Autodesk Inventor part; units mm, degrees
ref_plane "YZ Plane" through (0, 0, 0) normal (1, 0, 0) x (0, 1, 0)
ref_plane "XZ Plane" through (0, 0, 0) normal (0, 1, 0) x (-1, 0, 0)
ref_plane "XY Plane" through (0, 0, 0) normal (0, 0, 1) x (1, 0, 0)
sketch "Sketch1" plane through (0, 0, 0) normal (0, 0, 1) x (1, 0, 0)
  line L0 (0, 0) -> (35, 0)
  line L1 (35, 0) -> (35, 4.5)
  line L2 (35, 4.5) -> (4.5, 4.5)
  line L3 (4.5, 4.5) -> (4.5, 35)
  line L4 (4.5, 35) -> (0, 35)
  line L5 (0, 35) -> (0, 0)
  dimension "d0" = 35
  dimension "d1" = 35
  dimension "d2" = 4.5
  dimension "d3" = 4.5
extrude "Extrusion1" add sketch "Sketch1" along normal mid plane 28
sketch "Sketch2" plane through (0, 0, 14) normal (0, 0, 1) x (1, 0, 0)
  line L0 (0, 0) -> (35, 0)
  line L1 (35, 0) -> (35, 4.5)
  line L2 (35, 4.5) -> (4.5, 4.5)
  line L3 (4.5, 4.5) -> (4.5, 35)
  line L4 (4.5, 35) -> (0, 35)
  line L5 (0, 35) -> (0, 0)
  line L6 (4.5, 35) -> (6, 35)
  line L7 (6, 35) -> (6, 31)
  line L8 (6, 31) -> (31, 6)
  line L9 (31, 6) -> (35, 6)
  line L10 (35, 4.5) -> (4.5, 4.5)
  line L11 (35, 6) -> (35, 4.5)
  dimension "d6" = 45
  dimension "d7" = 1.5
  dimension "d8" = 1.5
  dimension "d9" = 4
extrude "Extrusion2" add sketch "Sketch2" against normal blind 2.8 contours L2 L3 L6 L7 L8 L9 L11
mirror "Mirror1" about plane through (0, 0, 0) normal (0, 0, 1) of "Extrusion2"
sketch "Sketch3" plane through (0, 0, 14) normal (-1, 0, 0) x (0, 0, 1)
  line L0 (0, 0) -> (-28, 0)
  line L1 (0, 35) -> (0, 0)
  line L2 (-28, 35) -> (0, 35)
  line L3 (-28, 0) -> (-28, 35)
  line L4 (-25.2, 35) -> (-2.8, 35) construction
  line L5 (-14, 35) -> (-14, 0) construction
  line L6 (-14, 21.5) -> (-14, 13.5)
  line L7 (-17.5, 21.5) -> (-17.5, 13.5)
  line L8 (-10.5, 13.5) -> (-10.5, 21.5)
  arc A0 (-10.5, 21.5) -> (-17.5, 21.5) centre (-14, 21.5) ccw
  arc A1 (-17.5, 13.5) -> (-10.5, 13.5) centre (-14, 13.5) ccw
  point P0 (-14, 17.5)
  point P1 (-14, 17.5)
  dimension "d12" = 8
  dimension "d13" = 3.5
extrude "Extrusion3" cut sketch "Sketch3" against normal through all contours A0 L8 A1 L7
sketch "Sketch4" plane through (0, 0, 14) normal (0, -1, 0) x (1, 0, 0)
  line L0 (35, -28) -> (35, 0)
  line L1 (0, 0) -> (35, 0)
  line L2 (0, 0) -> (0, -28)
  line L3 (35, -28) -> (0, -28)
  line L4 (0, -14) -> (35, -14) construction
  line L5 (13.5, -14) -> (21.5, -14) construction
  line L6 (13.5, -17.5) -> (21.5, -17.5)
  line L7 (21.5, -10.5) -> (13.5, -10.5)
  arc A0 (13.5, -10.5) -> (13.5, -17.5) centre (13.5, -14) ccw
  arc A1 (21.5, -17.5) -> (21.5, -10.5) centre (21.5, -14) ccw
  point P0 (17.5, -14)
  point P1 (17.5, -14)
  dimension "d16" = 8
  dimension "d17" = 3.5
extrude "Extrusion4" cut sketch "Sketch4" against normal through all contours A0 L7 A1 L6
properties part number "3030 Corner Bracket External"
Work out the finished part from the listing and answer in its coordinate system (mm). A direction names the side the tool comes from. Coordinates: 2 decimals unless noted, no trailing zeros. Loops run counter-clockwise (first coordinate to the right, second up) from the corner with the lowest first, then second, coordinate; pieces in that order, holes last. Notation, with made-up numbers: M 34.5,7.5 L 41.5,7.5 A13 ccw 41.5,25.5 Z; hole C 5.5,42 d4. An arc over 180 degrees is marked long. Answer in a Markdown table with one row per item. Add a question column.
1. Flat-ended cylindrical pins translate along their axes: P1, Ø2, axis at x = 34, z = -13, coming from the +Y side; P2, Ø2, axis at y = 34, z = 12, coming from the +X side; P3, Ø10, axis at x = 22, y = 26.5, coming from the +Z side; P4, Ø11, axis at x = 12.5, z = 1.5, coming from the +Y side. Find the tip coordinate at first contact, or state that the pin passes through.
2. Find section A-A, the plane y = 16. Write down the section's boundary in (x, z).
3. The mould has two halves that part along Z. Classify faces 1 (the flat face through (19, 18, -13)), 2 (the flat face through (13, 13, 11.2)), 3 (the flat face through (14, 14, -14)), 4 (the cylindrical face through (10, 2, 0)): pulls with the +Z half, pulls with the -Z half, needs draft (parallel to the pull), parting line crosses it, or undercut.
4. Consider L1, parallel to Z at x = 11, y = 21; L2, parallel to Z at x = 3.5, y = 20; L3, parallel to X at y = 17.5, z = -10.5. Determine where each line is inside the solid, lowest interval first.
5. Find section B-B, the plane z = -2.75. Write down the section's boundary in (x, y), then the cut area to 3 significant figures.
6. Find section D-D, the plane x = 24.5. Write down the section's boundary in (y, z), then the cut area to 3 significant figures.
7. Find section C-C, the plane y = 4. Write down the section's boundary in (x, z).
8. A tool of negligible diameter and unlimited length cuts with its end or side. For faces 5 (the flat face through (6, 33, 13)), 6 (the cylindrical face through (2, 10, 0)), 7 (the flat face through (4.5, 20, 5)), 8 (the flat face through (18, 2, 3.5)), from which of +Z, -Z, +X, -X, +Y, -Y can it reach the whole face along a straight path? Write none if from no direction.
Reported:
| question | item | result |
|---|---|---|
| 1 | P1 | stops at y = 6 |
| 1 | P2 | stops at x = 6 |
| 1 | P3 | passes through |
| 1 | P4 | stops at y = 4.5 |
| 2 | outline | M 0,-14 L 21,-14 L 21,-11.2 L 4.5,-11.2 L 4.5,-3.5 L 0,-3.5 Z; M 0,3.5 L 4.5,3.5 L 4.5,11.2 L 21,11.2 L 21,14 L 0,14 Z |
| 3 | face 1 | needs draft |
| 3 | face 2 | undercut |
| 3 | face 3 | pulls with the -Z half |
| 3 | face 4 | undercut |
| 4 | L1 | z = -14 to -11.2, 11.2 to 14 |
| 4 | L2 | z = -14 to -3.5, 3.5 to 14 |
| 4 | L3 | x = 0 to 4.5 |
| 5 | outline | M 0,0 L 11.33,0 L 11.33,4.5 L 4.5,4.5 L 4.5,11.33 L 0,11.33 Z; M 0,23.67 L 4.5,23.67 L 4.5,35 L 0,35 Z; M 23.67,0 L 35,0 L 35,4.5 L 23.67,4.5 Z |
| 5 | area | 184 mm^2 |
| 6 | outline | M 0,-14 L 12.5,-14 L 12.5,-11.2 L 4.5,-11.2 L 4.5,-1.8 L 0,-1.8 Z; M 0,1.8 L 4.5,1.8 L 4.5,11.2 L 12.5,11.2 L 12.5,14 L 0,14 Z |
| 6 | area | 155 mm^2 |
| 7 | outline | M 0,-14 L 35,-14 L 35,14 L 0,14 Z; hole M 13.5,-3.5 L 21.5,-3.5 A3.5 ccw 21.5,3.5 L 13.5,3.5 A3.5 ccw Z |
| 8 | face 5 | +Z, -Z, +X, +Y |
| 8 | face 6 | +X, -X |
| 8 | face 7 | +X, +Y |
| 8 | face 8 | +Y, -Y |
